For this review, take the finished solid that the model builds, in its own axes (mm). Face numbers are marked on the shaded views. A direction names the side the tool comes from. Coordinates: 2 decimals unless noted, no trailing zeros. Write each loop counter-clockwise with the first axis right and the second up, starting at its lowest first coordinate (ties: lowest second). Pieces come first, ordered by that corner, then holes.
```python
from build123d import *

# Parameters (mm, degrees)
F0_W      = 45
F0_H      = 14.9
F1_DEPTH  = 0.63
F2_R      = 7.4
F3_R      = 7.4
F4_DEPTH  = 0.63
F6_W      = 10
F6_H      = 40.06
F7_DEPTH  = 0.63
F8_DEPTH  = 0.63
F10_DEPTH = 0.05
F11_R     = 2.5
F13_DEPTH = 0.05
F15_D     = 2.7
F5_W      = 1.1
F5_H      = 1.1
F16_DEPTH = 0.631


with BuildPart() as f1:
    # F0 (on Top) → F1 (new body)
    with BuildSketch(Plane.XY):
        with Locations((-10.817694, -7.45)):
            Rectangle(F0_W, F0_H)
    extrude(amount=F1_DEPTH)

    # F2
    f2_edges = [f1.edges().sort_by_distance(p)[0] for p in [
        (-33.317694, 0, 0.315),
    ]]
    fillet(f2_edges, radius=F2_R)

    # F3
    f3_edges = [f1.edges().sort_by_distance(p)[0] for p in [
        (-33.317694, -14.9, 0.315),
    ]]
    fillet(f3_edges, radius=F3_R)

    # F0 (on Top) → F4 (join)
    with BuildSketch(Plane.XY):
        Polygon((11.682306, 24.95), (11.682306, 0), (11.682306, -14.9), (11.682306, -39.85), (22.972306, -39.85), (22.972306, 24.95), align=None)
    extrude(amount=F4_DEPTH)

    # F6 (on face) → F7 (join)
    with BuildSketch(Plane(origin=(11.682306, 0, 0), x_dir=(0, -1, 0), z_dir=(-1, 0, 0))):
        with Locations((34.85, 20.03)):
            Rectangle(F6_W, F6_H)
        with Locations((-19.95, 20.03)):
            Rectangle(F6_W, F6_H)
    extrude(amount=F7_DEPTH)

    # F6 (on face) → F8 (join)
    with BuildSketch(Plane(origin=(11.682306, 0, 0), x_dir=(0, -1, 0), z_dir=(-1, 0, 0))):
        with Locations((34.85, 20.03)):
            Rectangle(F6_W, F6_H)
        with BuildLine():
            Line((29.85, 40.06), (39.85, 40.06))
            ThreePointArc((39.85, 40.06), (7.45, 72.46), (-24.95, 40.06))
            Line((-24.95, 40.06), (-14.95, 40.06))
            ThreePointArc((-14.95, 40.06), (7.45, 62.46), (29.85, 40.06))
        make_face()
        with Locations((-19.95, 20.03)):
            Rectangle(F6_W, F6_H)
    extrude(amount=F8_DEPTH)

    # F9 (on face) → F10 (join, symmetric)
    with BuildSketch(Plane.XZ.offset(39.85)):
        with BuildLine():
            Line((11.682306, 36.690054), (11.682306, 0.63))
            Line((11.682306, 0.63), (19.082306, 0.63))
            Line((19.082306, 0.63), (19.082306, 10.063524))
            Line((19.082306, 10.063524), (13.692664, 38.690027))
            ThreePointArc((13.692664, 38.690027), (13.103211, 37.272156), (11.682306, 36.690054))
        make_face()
        with BuildLine():
            Line((11.682306, 40.06), (11.682306, 36.690054))
            ThreePointArc((11.682306, 36.690054), (13.103211, 37.272156), (13.692664, 38.690027))
            ThreePointArc((13.692664, 38.690027), (13.103211, 40.107898), (11.682306, 40.69))
            Line((11.682306, 40.69), (11.682306, 40.06))
        make_face()
    extrude(amount=F10_DEPTH, both=True)

    # F11
    f11_edges = [f1.edges().sort_by_distance(p)[0] for p in [
        (22.972306, -39.85, 0.315),
        (22.972306, 24.95, 0.315),
    ]]
    fillet(f11_edges, radius=F11_R)

    # F12 (on face) → F13 (join, symmetric)
    with BuildSketch(Plane(origin=(0, 24.95, 0), x_dir=(-1, 0, 0), z_dir=(0, 1, 0))):
        with BuildLine():
            Line((-18.452306, 7.854219), (-18.452306, 0.63))
            Line((-18.452306, 0.63), (-11.682306, 0.63))
            Line((-11.682306, 0.63), (-11.682306, 36.161817))
            ThreePointArc((-11.682306, 36.161817), (-12.762503, 37.023069), (-13.026688, 38.379087))
            Line((-13.026688, 38.379087), (-18.452306, 7.854219))
        make_face()
        with BuildLine():
            Line((-11.682306, 36.161817), (-11.682306, 39.958183))
            ThreePointArc((-11.682306, 39.958183), (-12.575161, 39.3565), (-13.026688, 38.379087))
            ThreePointArc((-13.026688, 38.379087), (-12.762503, 37.023069), (-11.682306, 36.161817))
        make_face()
    extrude(amount=F13_DEPTH, both=True)

    # F15 (through all)
    with Locations(Plane.YZ.offset(11.682306)):
        with Locations((-25.227612, 60.88687), (10.350126, 60.88687)):
            Hole(F15_D / 2)

    # F5 (on face) → F16 (cut, through all)
    with BuildSketch(Plane.XY.offset(0.63)):
        with Locations((12.232306, 24.4)):
            Rectangle(F5_W, F5_H)
        with BuildLine():
            ThreePointArc((11.682306, 0), (13.032306, 1.35), (11.682306, 2.7))
            Line((11.682306, 2.7), (11.682306, 0))
        make_face()
        with BuildLine():
            Line((11.682306, -14.9), (11.682306, -17.6))
            ThreePointArc((11.682306, -17.6), (13.032306, -16.25), (11.682306, -14.9))
        make_face()
        with Locations((12.232306, -39.3)):
            Rectangle(F5_W, F5_H)
    extrude(amount=-F16_DEPTH, mode=Mode.SUBTRACT)


solid = f1.part
```
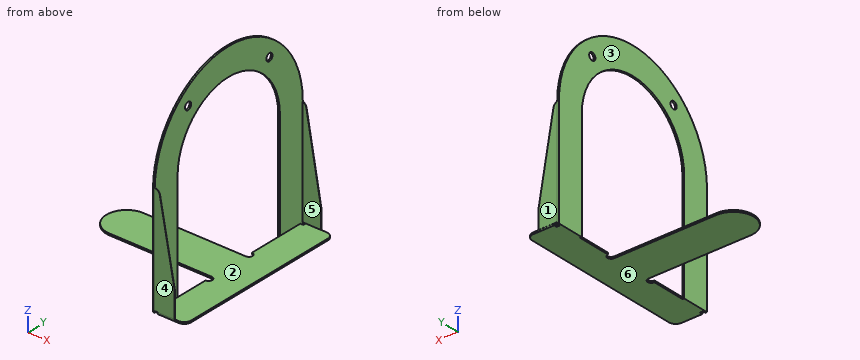
1) Consider section A-A (y = -27.5). Give the boundary of the cut face in (x, z).
2) The part is to be moulded in two halves that separate along Y. For the marked faces 1, 2, 3 and 4, say which applies: pulls with the +Y half, pulls with the -Y half, needs draft (parallel to the pull), parting line crosses it, or undercut.
3) Tool access review of the marked faces 5 and 6: name each direction out of +Z, -Z, +X, -X, +Y, -Y from which nothing blocks a thin tool from reaching the whole face with its end or side.
4) Consider section D-D (z = 9). Give the boundary of the cut face in (x, y).
5) For L1, parallel to X at y = -31.5, z = 34.5; L2, parallel to Z at x = -9, y = -6, list the stretches that pass through material, from the lowest coordinate up.
6) Clearance check with flat-ended pins moving along their axes: P1, Ø10, axis at x = 10.5, y = -0.5, coming from the +Z side; P2, Ø0.7, axis at x = -13, z = 0.5, coming from the -Y side; P3, Ø0.5, axis at y = 24.5, z = 0, coming from the -X side; P4, Ø1, axis at x = -23, y = 2, coming from the +Z side. State where each tip first meets the part, or that it passes through.
7) Consider section B-B (z = 18.5). Give the boundary of the cut face in (x, y), then the cut area to 3 significant figures.
8) Consider section C-C (x = -16.5). Give the boundary of the cut face in (y, z), then the cut area to 3 significant figures.
Results:
1. outline: (11.05, 50.05) - (11.68, 50.05) - (11.68, 65.51) - (11.05, 65.51) - close; (11.68, 0) - (22.97, 0) - (22.97, 0.63) - (11.68, 0.63) - close
2. face 1: pulls with the +Y half
2. face 2: undercut
2. face 3: needs draft
2. face 4: pulls with the -Y half
3. face 5: +Z, +X
3. face 6: -Z, +X, -X, +Y, -Y
4. outline: (11.05, -39.85) - (11.68, -39.85) - (11.68, -39.9) - (19.08, -39.9) - (19.08, -39.8) - (11.68, -39.8) - (11.68, -29.85) - (11.05, -29.85) - close; (11.05, 14.95) - (11.68, 14.95) - (11.68, 24.9) - (18.25, 24.9) - (18.25, 25) - (11.68, 25) - (11.68, 24.95) - (11.05, 24.95) - close
5. L1: x = 11.05 to 11.68
5. L2: z = 0 to 0.63
6. P1: stops at z = 72.4
6. P2: stops at y = -14.9
6. P3: stops at x = 11.05
6. P4: passes through
7. outline: (11.05, -39.85) - (11.68, -39.85) - (11.68, -39.9) - (17.49, -39.9) - (17.49, -39.8) - (11.68, -39.8) - (11.68, -29.85) - (11.05, -29.85) - close; (11.05, 14.95) - (11.68, 14.95) - (11.68, 24.9) - (16.56, 24.9) - (16.56, 25) - (11.68, 25) - (11.68, 24.95) - (11.05, 24.95) - close
7. area: 13.7 mm2
8. outline: (-14.9, 0) - (0, 0) - (0, 0.63) - (-14.9, 0.63) - close
8. area: 9.39 mm2
